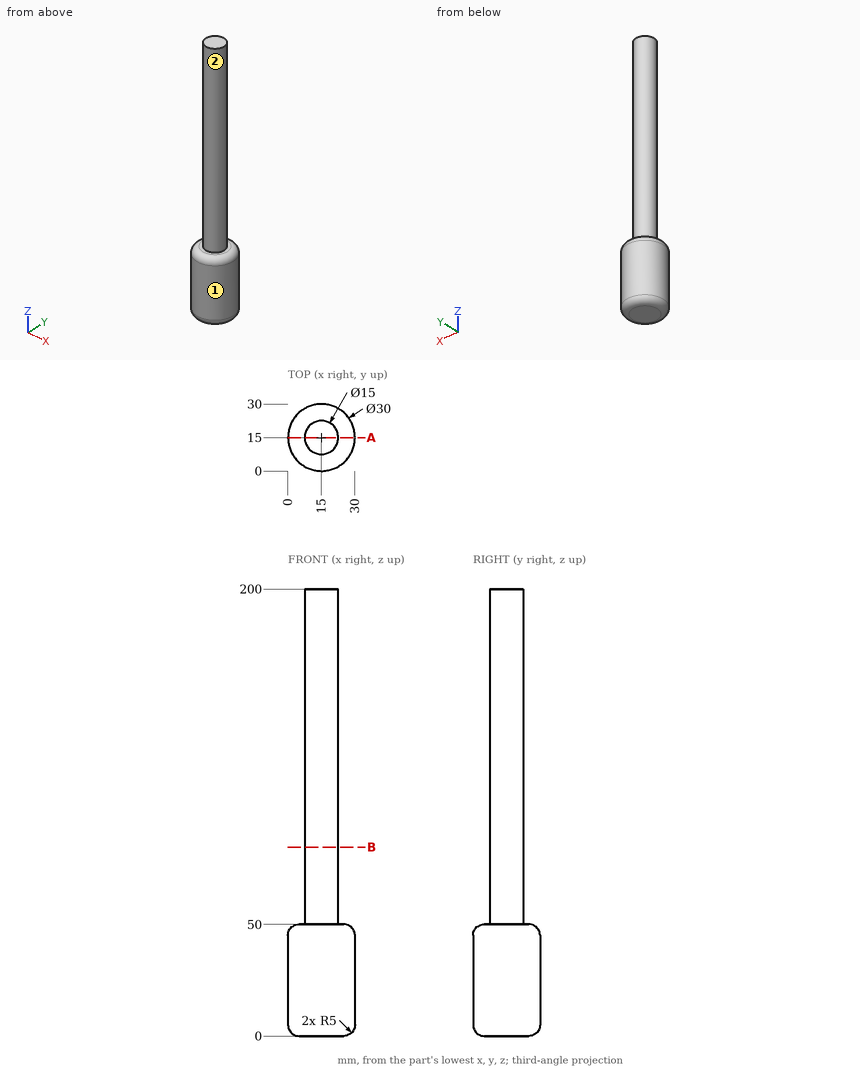
Geometry: see drawing. Coordinates: mm, zero at the bounding-box minimum. A direction names the side the tool comes from. Coordinates: 2 decimals unless noted, no trailing zeros. Order: outer loops, then holes, each group sorted by start corner. A loop starts at its lowest first (then second) coordinate and runs counter-clockwise, first axis right, second up. Notation, with made-up numbers: (1, -10.75) -> (5, -10.75) arc R17 cw to (5, 4.25) -> close; hole circle Ø7 at (-3, 38.5). An arc over 180 degrees is marked (long way). Write each question's results on one line, items separated by ' | '. Start each with the question number.
1) Set-up query: the marked faces 1 and 2. Return all of +Z, -Z, +X, -X, +Y, -Y with unobstructed straight access to the full face (end or side cutting, diameter ignored); none if empty.
2) First-contact query: pin 1 (8 mm diameter, centred on x = 19.5, z = 171, fed in from +Y); pin 2 (5 mm diameter, centred on x = 12.5, z = 76, fed in from -Y); pin 3 (12 mm diameter, centred on x = 7, z = 43.5, fed in from -Y). Flat tips, straight axial feed; report the tip coordinate or a pass-through.
3) Cut plane B-B, the plane z = 84.5. Output: boundary loops of the cut face in (x, y).
4) Cut plane A-A, the plane y = 15. Output: boundary loops of the cut face in (x, z), and give its area (3 significant figures).
5) Material intervals for line 1 along Y through (x, z) = (15, 99); line 2 along Z through (x, y) = (7, 17.5); line 3 along Y through (x, z) = (13, 131), sorted ascending.
Checks:
1) face 1: +Z, -Z | face 2: +Z
2) pin 1: y = 22.48 | pin 2: y = 7.5 | pin 3: y = 0.13
3) outline: circle Ø15 at (15, 15)
4) outline: (0, 5) arc R5 ccw to (5, 0) -> (25, 0) arc R5 ccw to (30, 5) -> (30, 45) arc R5 ccw to (25, 50) -> (22.5, 50) -> (22.5, 200) -> (7.5, 200) -> (7.5, 50) -> (5, 50) arc R5 ccw to (0, 45) -> close | area: 3,730 mm^2
5) line 1: 7.5 to 22.5 | line 2: 0 to 50 | line 3: 7.77 to 22.23
